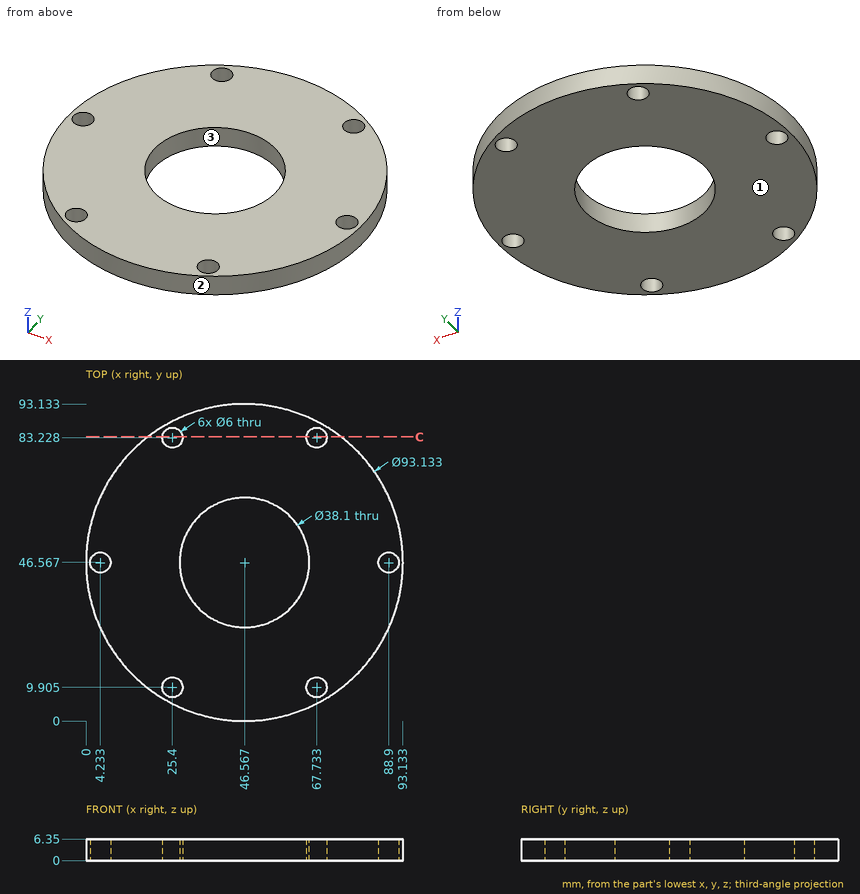
Part print with two shaded views. Sizes in mm from the minimum x, y, z corner. Coordinates: 2 decimals unless noted, no trailing zeros.
(1) Cut at C-C on y = 83.5. State how many separate pieces and enclosed holes the cut face has, and give its area (3 significant figures).
(2) Mould opens along Y. For the marked faces 1, 2 and 3 say: pulls with the +Y half, pulls with the -Y half, needs draft (parallel to the pull), parting line crosses it, or undercut.
(3) Drill centre lines: line 1 (Y direction, x = 25.4, z = 2) (1 decimal); line 2 (X direction, y = 9.5, z = 1) (1 decimal); line 3 (Y direction, x = 34.5, z = 2.5) (1 decimal). Where is each one in solid material? Low to high.
(4) Pin check, flat tips, straight feed: pin 1 Ø5 at (x, y) = (25.4, 83.23) entering from +Z; pin 2 Ø3 at (x, z) = (16.5, 5) entering from -Y; pin 3 Ø2 at (x, z) = (44.5, 4) entering from -Y; pin 4 Ø1 at (y, z) = (11.5, 1.5) entering from -X (1 decimal). Stop position of each tip, or through.
Working result:
1. separate pieces: 3
1. enclosed holes: 0
1. area: 284 mm2
2. face 1: needs draft
2. face 2: parting line crosses it
2. face 3: undercut
3. line 1: y = 5.1 to 6.9, 12.9 to 80.2, 86.2 to 88
3. line 2: x = 18.4 to 22.4, 28.4 to 64.8, 70.7 to 74.8
3. line 3: y = 1.6 to 31.8, 61.3 to 91.5
4. pin 1: passes through
4. pin 2: stops at y = 9.79
4. pin 3: stops at y = 0.01
4. pin 4: stops at x = 15.4
